from build123d import *

# Parameters (mm, degrees)
SKETCH1_R           = 1.65
SKETCH1_R_2         = 6.15
BOSS_EXTRUDE1_DEPTH = 72
CUT_EXTRUDE1_DEPTH  = 57
SKETCH3_R           = 1.5
CUT_EXTRUDE2_DEPTH  = 92.028841583
SKETCH4_W           = 24
SKETCH4_H           = 72
SKETCH4_R           = 1.5
BOSS_EXTRUDE2_DEPTH = 3
FILLET1_R           = 6


with BuildPart() as part:
    # Sketch1 → Boss-Extrude1 (new body)
    with BuildSketch(Plane.XY):
        with BuildLine():
            Line((-21, 0), (-21, -21.5))
            Line((-21, -21.5), (-36, -21.5))
            Line((-36, -21.5), (-36, -24.5))
            Line((-36, -24.5), (36, -24.5))
            Line((36, -24.5), (36, -21.5))
            Line((36, -21.5), (21, -21.5))
            Line((21, -21.5), (21, 0))
            ThreePointArc((21, 0), (0, 21), (-21, 0))
        make_face()
        with Locations((0, 15.5)):
            Circle(SKETCH1_R, mode=Mode.SUBTRACT)
        with Locations((13.423393759, 7.75)):
            Circle(SKETCH1_R, mode=Mode.SUBTRACT)
        with Locations((13.423393759, -7.75)):
            Circle(SKETCH1_R, mode=Mode.SUBTRACT)
        with Locations((0, -15.5)):
            Circle(SKETCH1_R, mode=Mode.SUBTRACT)
        with Locations((-13.423393759, -7.75)):
            Circle(SKETCH1_R, mode=Mode.SUBTRACT)
        with Locations((-13.423393759, 7.75)):
            Circle(SKETCH1_R, mode=Mode.SUBTRACT)
        with Locations((7, 0)):
            Circle(SKETCH1_R_2, mode=Mode.SUBTRACT)
    extrude(amount=BOSS_EXTRUDE1_DEPTH)

    # Sketch2 → Cut-Extrude1 (cut)
    with BuildSketch(Plane.XY.offset(72)):
        with BuildLine():
            Line((-18.5, 0), (-18.5, -21.5))
            Line((-18.5, -21.5), (18.5, -21.5))
            Line((18.5, -21.5), (18.5, 0))
            ThreePointArc((18.5, 0), (0, 18.5), (-18.5, 0))
        make_face()
    extrude(amount=-CUT_EXTRUDE1_DEPTH, mode=Mode.SUBTRACT)

    # Sketch3 → Cut-Extrude2 (cut, through all)
    with BuildSketch(Plane(origin=(0, -21.5, 0), x_dir=(1, 0, 0), z_dir=(0, 1, 0))):
        with Locations(Location((-28.5, -36, 0), (0, 0, 270))):
            Circle(SKETCH3_R)
        with Locations(Location((-28.5, -6, 0), (0, 0, 270))):
            Circle(SKETCH3_R)
        with Locations(Location((-28.5, -66, 0), (0, 0, 270))):
            Circle(SKETCH3_R)
        with Locations(Location((28.5, -66, 0), (0, 0, 90))):
            Circle(SKETCH3_R)
        with Locations(Location((28.5, -6, 0), (0, 0, 90))):
            Circle(SKETCH3_R)
        with Locations(Location((28.5, -36, 0), (0, 0, 90))):
            Circle(SKETCH3_R)
    extrude(amount=-CUT_EXTRUDE2_DEPTH, mode=Mode.SUBTRACT)

    # Sketch4 → Boss-Extrude2 (add)
    with BuildSketch(Plane(origin=(0, -21.5, 0), x_dir=(1, 0, 0), z_dir=(0, 1, 0))):
        with Locations((48, -36)):
            Rectangle(SKETCH4_W, SKETCH4_H)
        with Locations(Location((48, -10.5, 0), (0, 0, 270))):
            Circle(SKETCH4_R, mode=Mode.SUBTRACT)
        with Locations(Location((48, -46.5, 0), (0, 0, 270))):
            Circle(SKETCH4_R, mode=Mode.SUBTRACT)
    extrude(amount=-BOSS_EXTRUDE2_DEPTH)

    # Fillet1
    fillet1_edges = [part.edges().sort_by_distance(p)[0] for p in [
        (60, -23, 0),
    ]]
    fillet(fillet1_edges, radius=FILLET1_R)


solid = part.part
Build history of the part. All positions in model axes, mm. A direction names the side the tool comes from. Coordinates: 2 decimals unless noted, no trailing zeros. Write each loop counter-clockwise with the first axis right and the second up, starting at its lowest first coordinate (ties: lowest second). Pieces come first, ordered by that corner, then holes.
(1) Drill centre lines: line 1 (X direction, y = -7.75, z = 6.75); line 2 (X direction, y = -22.35, z = 66); line 3 (X direction, y = -2, z = 23.5). Where is each one in solid material? Low to high.
(2) Cut at C-C on x = 28.5. List the corners of the cut face in (y, z), and give its area (3 significant figures).
(3) Mould opens along X. For faces 1 (the flat face through (-27, -21.5, 35)), 2 (the cylindrical face through (-27.235, -22.979, 66.806)), 3 (the flat face through (21, -11, 35)) say: pulls with the +X half, pulls with the -X half, needs draft (parallel to the pull), parting line crosses it, or undercut.
(4) Cut at B-B on y = -7.75. List the corners of the cut face in (x, z), and give its area (3 significant figures).
(5) Pin check, flat tips, straight feed: pin 1 Ø2.5 at (x, z) = (28.5, 36) entering from +Y; pin 2 Ø6.5 at (y, z) = (-11.5, 35.5) entering from -X; pin 3 Ø11 at (y, z) = (-12.5, 31.5) entering from +X; pin 4 Ø3 at (y, z) = (7, 10) entering from -X. Stop position of each tip, or through.
(6) 3-axis set-ups, long thin cutter, end or side, ignore diameter. For faces 4 (the cylindrical face through (-11.9, -8.38, 7.4)), 5 (the cylindrical face through (0.407, 18.496, 43.899)): which of +Z, -Z, +X, -X, +Y, -Y reach the whole face in a straight line?
(7) Cut at D-D on z = 46.5. List the corners of the cut face in (x, y).
(8) Cut at A-A on z = 66. List the corners of the cut face in (x, y).
Working result:
1. line 1: x = -21 to -15.07, -11.77 to 11.77, 15.07 to 21
1. line 2: x = -36 to -30, -27 to 27, 30 to 60
1. line 3: x = -21 to -18.5, 18.5 to 21
2. outline: (-24.5, 0) - (-21.5, 0) - (-21.5, 4.5) - (-24.5, 4.5) - close; (-24.5, 7.5) - (-21.5, 7.5) - (-21.5, 34.5) - (-24.5, 34.5) - close; (-24.5, 37.5) - (-21.5, 37.5) - (-21.5, 64.5) - (-24.5, 64.5) - close; (-24.5, 67.5) - (-21.5, 67.5) - (-21.5, 72) - (-24.5, 72) - close
2. area: 189 mm2
3. face 1: needs draft
3. face 2: undercut
3. face 3: pulls with the +X half
4. outline: (-21, 0) - (-15.07, 0) - (-15.07, 15) - (-18.5, 15) - (-18.5, 72) - (-21, 72) - close; (-11.77, 0) - (11.77, 0) - (11.77, 15) - (-11.77, 15) - close; (15.07, 0) - (21, 0) - (21, 72) - (18.5, 72) - (18.5, 15) - (15.07, 15) - close
4. area: 816 mm2
5. pin 1: passes through
5. pin 2: stops at x = -21
5. pin 3: stops at x = 21
5. pin 4: stops at x = -20.27
6. face 4: +Z, -Z
6. face 5: +Z
7. outline: (-36, -24.5) - (46.5, -24.5) - (46.5, -21.5) - (21, -21.5) - (21, 0) arc R21 ccw to (-21, 0) - (-21, -21.5) - (-36, -21.5) - close; (49.5, -24.5) - (60, -24.5) - (60, -21.5) - (49.5, -21.5) - close; hole (-18.5, -21.5) - (18.5, -21.5) - (18.5, 0) arc R18.5 ccw to (-18.5, 0) - close
8. outline: (-36, -24.5) - (-30, -24.5) - (-30, -21.5) - (-36, -21.5) - close; (-27, -24.5) - (27, -24.5) - (27, -21.5) - (21, -21.5) - (21, 0) arc R21 ccw to (-21, 0) - (-21, -21.5) - (-27, -21.5) - close; (30, -24.5) - (60, -24.5) - (60, -21.5) - (30, -21.5) - close; hole (-18.5, -21.5) - (18.5, -21.5) - (18.5, 0) arc R18.5 ccw to (-18.5, 0) - close
